```python
from build123d import *

# Parameters (mm, degrees)
SKETCH1_W                  = 298.45
SKETCH1_H                  = 495.3
BOSS_EXTRUDE1_DEPTH        = 4.7625
CUT_EXTRUDE1_DEPTH         = 290.291114191
CUT_EXTRUDE1_DEPTH_BACK    = 290.291114191
SKETCH3_W                  = 196.85
SKETCH3_H                  = 114.3
SKETCH20_W                 = 47.879
SKETCH20_H                 = 47.879
CUT_EXTRUDE5_DEPTH         = 290.291114191
F_10_CLEARANCE_HOLE1_D     = 5.1054
F_10_CLEARANCE_HOLE1_DEPTH = 10.668
F_10_CLEARANCE_HOLE1_TIP   = 1.533816902
F_10_CLEARANCE_HOLE4_D     = 5.1054
LPATTERN3_COUNT            = 3
LPATTERN3_PITCH            = 63.5
MIRROR2_COPY_1_D           = 5.1054
MIRROR2_COPY_2_D           = 5.1054
F_10_CLEARANCE_HOLE5_D     = 5.1054
LPATTERN4_COUNT            = 3
LPATTERN4_PITCH            = 96.52
LPATTERN4_COL_COUNT        = 3
LPATTERN4_COL_PITCH        = 96.52
MIRROR3_COPY_1_D           = 5.1054
MIRROR3_COPY_2_D           = 5.1054
MIRROR3_COPY_3_D           = 5.1054
MIRROR3_COPY_4_D           = 5.1054
F_10_CLEARANCE_HOLE6_D     = 5.1054
F_10_CLEARANCE_HOLE7_D     = 5.1054
F_10_CLEARANCE_HOLE8_D     = 5.1054


with BuildPart() as part:
    # Sketch1 → Boss-Extrude1 (new, symmetric)
    with BuildSketch(Plane(origin=(0, 0, 0), x_dir=(1, 0, 0), z_dir=(0, 1, 0))):
        Rectangle(SKETCH1_W, SKETCH1_H)
    extrude(amount=BOSS_EXTRUDE1_DEPTH, both=True)

    # Sketch3 → Cut-Extrude1 (cut, two sides: drawn at the far end of the back side and taken through both)
    with BuildSketch(Plane(origin=(0, 4.7625, 0), x_dir=(1, 0, 0), z_dir=(0, 1, 0)).offset(-CUT_EXTRUDE1_DEPTH_BACK)):
        with Locations((0, -44.45)):
            Rectangle(SKETCH3_W, SKETCH3_H)
    extrude(amount=CUT_EXTRUDE1_DEPTH + CUT_EXTRUDE1_DEPTH_BACK, mode=Mode.SUBTRACT)

    # Sketch20 → Cut-Extrude5 (cut, through all)
    with BuildSketch(Plane.XZ.offset(4.7625)):
        with Locations((0, 171.45)):
            Rectangle(SKETCH20_W, SKETCH20_H)
    extrude(amount=-CUT_EXTRUDE5_DEPTH, mode=Mode.SUBTRACT)

    # #10 Clearance Hole1
    with Locations(Plane(origin=(0, -4.7625, 0), x_dir=(-1, 0, 0), z_dir=(0, -1, 0))):
        with Locations((-38.1, -155.575), (38.1, -155.575), (38.1, -187.325), (-38.1, -187.325)):
            Hole(F_10_CLEARANCE_HOLE1_D / 2, depth=F_10_CLEARANCE_HOLE1_DEPTH)
            with Locations((0, 0, -(F_10_CLEARANCE_HOLE1_DEPTH + F_10_CLEARANCE_HOLE1_TIP / 2))):  # 118° drill point
                Cone(0, F_10_CLEARANCE_HOLE1_D / 2, F_10_CLEARANCE_HOLE1_TIP, mode=Mode.SUBTRACT)

    # #10 Clearance Hole4 (through all)
    with Locations(Plane(origin=(0, 4.7625, 0), x_dir=(1, 0, 0), z_dir=(0, 1, 0))):
        with Locations((-63.5, 241.3)):
            f_10_clearance_hole4 = Hole(F_10_CLEARANCE_HOLE4_D / 2)

    # LPattern3: #10 Clearance Hole4 ×3
    with Locations(*[(i * LPATTERN3_PITCH, 0, 0) for i in range(1, LPATTERN3_COUNT)]):
        add(f_10_clearance_hole4, mode=Mode.SUBTRACT)

    # Mirror2: #10 Clearance Hole4 across plane
    add(f_10_clearance_hole4.mirror(Plane.XY), mode=Mode.SUBTRACT)

    # Mirror2 copy 1 (through all)
    with Locations(Plane(origin=(63.5, 4.7625, 0), x_dir=(1, 0, 0), z_dir=(0, 1, 0))):
        with Locations((-63.5, -241.3)):
            Hole(MIRROR2_COPY_1_D / 2)

    # Mirror2 copy 2 (through all)
    with Locations(Plane(origin=(127, 4.7625, 0), x_dir=(1, 0, 0), z_dir=(0, 1, 0))):
        with Locations((-63.5, -241.3)):
            Hole(MIRROR2_COPY_2_D / 2)

    # #10 Clearance Hole5 (through all)
    with Locations(Plane(origin=(0, 4.7625, 0), x_dir=(1, 0, 0), z_dir=(0, 1, 0))):
        with Locations((-142.875, 0)):
            f_10_clearance_hole5 = Hole(F_10_CLEARANCE_HOLE5_D / 2)

    # LPattern4: #10 Clearance Hole5 ×3
    with Locations(*[(0, 0, -i * LPATTERN4_PITCH) for i in range(1, LPATTERN4_COUNT)]):
        add(f_10_clearance_hole5, mode=Mode.SUBTRACT)

    # LPattern4 col: #10 Clearance Hole5 ×3
    with Locations(*[(0, 0, i * LPATTERN4_COL_PITCH) for i in range(1, LPATTERN4_COL_COUNT)]):
        add(f_10_clearance_hole5, mode=Mode.SUBTRACT)

    # Mirror3: #10 Clearance Hole5 across plane
    add(f_10_clearance_hole5.mirror(Plane(origin=(0, 0, 0), x_dir=(0, 0, 1), z_dir=(1, 0, 0))), mode=Mode.SUBTRACT)

    # Mirror3 copy 1 (through all)
    with Locations(Plane(origin=(0, 4.7625, -96.52), x_dir=(-1, 0, 0), z_dir=(0, 1, 0))):
        with Locations((-142.875, 0)):
            Hole(MIRROR3_COPY_1_D / 2)

    # Mirror3 copy 2 (through all)
    with Locations(Plane(origin=(0, 4.7625, -193.04), x_dir=(-1, 0, 0), z_dir=(0, 1, 0))):
        with Locations((-142.875, 0)):
            Hole(MIRROR3_COPY_2_D / 2)

    # Mirror3 copy 3 (through all)
    with Locations(Plane(origin=(0, 4.7625, 96.52), x_dir=(-1, 0, 0), z_dir=(0, 1, 0))):
        with Locations((-142.875, 0)):
            Hole(MIRROR3_COPY_3_D / 2)

    # Mirror3 copy 4 (through all)
    with Locations(Plane(origin=(0, 4.7625, 193.04), x_dir=(-1, 0, 0), z_dir=(0, 1, 0))):
        with Locations((-142.875, 0)):
            Hole(MIRROR3_COPY_4_D / 2)

    # #10 Clearance Hole6 (through all)
    with Locations(Plane(origin=(0, 4.7625, 0), x_dir=(1, 0, 0), z_dir=(0, 1, 0))):
        with Locations((120.65, 32.5755), (120.65, -121.4755), (-120.65, -121.4755), (-120.65, 32.5755)):
            Hole(F_10_CLEARANCE_HOLE6_D / 2)

    # #10 Clearance Hole7 (through all)
    with Locations(Plane(origin=(0, 4.7625, 0), x_dir=(1, 0, 0), z_dir=(0, 1, 0))):
        with Locations((76.2, 32.5755), (0, 32.5755), (-76.2, 32.5755), (76.2, -121.4755), (0, -121.4755), (-76.2, -121.4755)):
            Hole(F_10_CLEARANCE_HOLE7_D / 2)

    # #10 Clearance Hole8 (through all)
    with Locations(Plane(origin=(0, 4.7625, 0), x_dir=(1, 0, 0), z_dir=(0, 1, 0))):
        with Locations((-142.875, -71.12), (142.875, -25.4), (-142.875, -25.4), (142.875, -71.12)):
            Hole(F_10_CLEARANCE_HOLE8_D / 2)


solid = part.part
```
The listing builds one solid part. Answer for the finished solid, in the listing's coordinates (mm). A direction names the side the tool comes from. Give positions to 0.01 mm unless a question says otherwise; leave off trailing zeros. Loops run counter-clockwise (first coordinate to the right, second up) from the corner with the lowest first, then second, coordinate; pieces in that order, holes last. Notation, with made-up numbers: (14, 16) - (56, 16) arc R24 cw to (56, 34) - close; hole circle Ø9 at (82.5, -28.5). An arc over 180 degrees is marked (long way). Return JSON: item names as keys, results as strings. Group by question number.
1. Determine the mould class of faces 1 (the flat face through (-2, 0, 247.65)), 2 (the flat face through (-23.94, 0, 171)), 3 (the flat face through (-2, -4.762, -59)) for opening direction Z: pulls with the +Z half, pulls with the -Z half, needs draft (parallel to the pull), parting line crosses it, or undercut.
2. Find section B-B (y = -2). State how many separate pieces and enclosed holes the cut face has, then the cut area to 3 significant figures.
3. Straight lines are drawn through the part: line 1 (Z direction, x = -76.2, y = 2.5); line 2 (Z direction, x = -38.1, y = -1); line 3 (X direction, y = 0.5, z = -241.3) (3 decimals). For each, find the intervals that lie inside material, in ascending order. Write a range as [from, to].
4. Given pin 1 Ø4.5 at (x, z) = (-142.875, 0) entering from -Y, flat-ended and moving along its own axis, determine where the tip first touches the part or whether it passes through.
5. Which of the six approach directions +Z, -Z, +X, -X, +Y, -Y give full straight-line access (tool end or side, diameter ignored) to faces 4 (the flat face through (-2, 4.762, -59)), 5 (the flat face through (98.425, 0, 45))?
6. Find section A-A (x = 45.5). Write down the section's boundary in (y, z).
Verdict:
{
 "1": {"face 1": "pulls with the +Z half", "face 2": "undercut", "face 3": "needs draft"},
 "2": {"separate pieces": "1", "enclosed holes": "36", "area": "122,000 mm^2"},
 "3": {"line 1": "z = [-247.65, -35.13], [-30.02, -12.7], [101.6, 118.92], [124.03, 247.65]", "line 2": "z = [-247.65, -12.7], [101.6, 153.02], [158.13, 184.77], [189.88, 247.65]", "line 3": "x = [-149.225, -66.053], [-60.947, -2.553], [2.553, 60.947], [66.053, 149.225]"},
 "4": {"pin 1": "passes through"},
 "5": {"face 4": "+Z, -Z, +X, -X, +Y", "face 5": "+Y, -Y"},
 "6": {"outline": "(-4.76, -247.65) - (4.76, -247.65) - (4.76, -12.7) - (-4.76, -12.7) - close; (-4.76, 101.6) - (4.76, 101.6) - (4.76, 247.65) - (-4.76, 247.65) - close"}
}
